Autodesk Inventor part; units mm, degrees
ref_plane "YZ Plane" through (0, 0, 0) normal (1, 0, 0) x (0, 1, 0)
ref_plane "XZ Plane" through (0, 0, 0) normal (0, 1, 0) x (-1, 0, 0)
ref_plane "XY Plane" through (0, 0, 0) normal (0, 0, 1) x (1, 0, 0)
sketch "Sketch1" plane through (0, 0, 0) normal (0, 0, 1) x (1, 0, 0)
  line L0 (-68.58, -128.7145) -> (68.58, -128.7145)
  line L1 (68.58, -128.7145) -> (68.58, 128.7145)
  line L2 (68.58, 128.7145) -> (-68.58, 128.7145)
  line L3 (-68.58, 128.7145) -> (-68.58, -128.7145)
  line L4 (-68.58, -128.7145) -> (68.58, 128.7145) construction
  line L5 (68.58, -128.7145) -> (-68.58, 128.7145) construction
  point P0 (0, 0)
  dimension "d0" = 137.16
  dimension "d1" = 257.429
extrude "Extrusion1" add sketch "Sketch1" against normal blind 3.175
sketch "Sketch2" plane through (0, 0, 0) normal (0, 0, 1) x (1, 0, 0)
  circle A0 centre (-59.69, 52.5145) radius 2.0955
  line L0 (-68.58, 128.7145) -> (-68.58, -128.7145)
  line L1 (-68.58, 128.7145) -> (68.58, 128.7145)
  circle A1 centre (59.69, 52.5145) radius 2.0955
  line L2 (68.58, -128.7145) -> (68.58, 128.7145)
  circle A2 centre (-59.69, -116.0145) radius 2.0955
  circle A3 centre (59.69, -116.0145) radius 2.0955
  line L3 (-68.58, -128.7145) -> (68.58, -128.7145)
  point P0 (0, 0)
  dimension "d4" = 8.89
  dimension "d5" = 76.2
  dimension "d6" = 76.2
  dimension "d7" = 8.89
  dimension "d8" = 4.191
  dimension "d9" = 12.7
  dimension "d10" = 8.89
  dimension "d11" = 8.89
  dimension "d12" = 12.7
  dimension "d13" = 4.191
  dimension "d21" = 4.191
  dimension "d22" = 4.191
hole "Hole1" at (-59.69, 52.5145, 0) at (59.69, 52.5145, 0) at (-59.69, -116.0145, 0) at (59.69, -116.0145, 0) direction (0, 0, -1) diameter 4.191 end through all
sketch "Sketch4" plane through (0, 0, 0) normal (0, 0, 1) x (1, 0, 0)
  line L0 (-35.179, -49.0855) -> (-35.179, -99.8855)
  line L1 (-28.321, -49.0855) -> (-28.321, -99.8855)
  line L2 (28.321, -49.0855) -> (28.321, -99.8855)
  line L3 (35.179, -49.0855) -> (35.179, -99.8855)
  line L4 (-68.58, 128.7145) -> (-68.58, -128.7145)
  line L5 (68.58, -128.7145) -> (68.58, 128.7145)
  line L6 (-68.58, -128.7145) -> (68.58, -128.7145)
  arc A0 (-28.321, -49.0855) -> (-35.179, -49.0855) centre (-31.75, -49.0855) ccw
  arc A1 (-35.179, -99.8855) -> (-28.321, -99.8855) centre (-31.75, -99.8855) ccw
  arc A2 (35.179, -49.0855) -> (28.321, -49.0855) centre (31.75, -49.0855) ccw
  arc A3 (28.321, -99.8855) -> (35.179, -99.8855) centre (31.75, -99.8855) ccw
  point P0 (0, 0)
  dimension "d23" = 6.858
  dimension "d24" = 6.858
  dimension "d25" = 33.401
  dimension "d26" = 50.8
  dimension "d27" = 33.401
  dimension "d28" = 28.829
  dimension "d29" = 28.829
  dimension "d30" = 28.829
  dimension "d31" = 28.829
  dimension "d32" = 50.8
  dimension "d33" = 50.8
  dimension "d34" = 50.8
extrude "Extrusion2" cut sketch "Sketch4" against normal blind 3.175
sketch "Sketch5" plane through (0, 0, 0) normal (0, 0, 1) x (1, 0, 0)
  line L0 (-68.58, 128.7145) -> (68.58, 128.7145)
  line L1 (68.58, 128.7145) -> (68.58, -128.7145)
  point P0 (0, 0)
  point P1 (-43.3324, 96.9645)
  point P2 (43.3324, 96.9645)
  dimension "d37" = 31.75
  dimension "d38" = 86.6648
  dimension "d39" = 31.75
  dimension "d40" = 25.2476
hole "Hole2" at (-43.3324, 96.9645, 0) at (43.3324, 96.9645, 0) direction (0, 0, -1) diameter 4.4704 end through all
sketch "battery_buzzer" plane through (0, 0, 0) normal (0, 0, 1) x (1, 0, 0)
  point P0 (0, 0)
sketch "Sketch10" plane through (0, 0, 0) normal (0, 0, 1) x (1, 0, 0)
  line L0 (-50.8, -128.7145) -> (-50.8, 39.8145)
  line L1 (-50.8, 39.8145) -> (50.8, 39.8145)
  line L2 (50.8, 39.8145) -> (50.8, -128.7145)
  line L3 (68.58, 128.7145) -> (-68.58, 128.7145)
  line L4 (-68.58, 128.7145) -> (-68.58, -128.7145)
  line L5 (68.58, 128.7145) -> (68.58, -128.7145)
  line L6 (-50.8, -128.7145) -> (50.8, -128.7145)
  point P0 (0, 0)
  dimension "d48" = 88.9
  dimension "d49" = 17.78
  dimension "d50" = 17.78
extrude "Extrusion3" cut sketch "Sketch10" against normal blind 3.175
CAD build for the part. Positions are in the model's coordinates, mm. Coordinates: 2 decimals unless noted, no trailing zeros. Write each loop counter-clockwise with the first axis right and the second up, starting at its lowest first coordinate (ties: lowest second). Pieces come first, ordered by that corner, then holes. Notation, with made-up numbers: M 80,63 L 130,63 A18 ccw 130,81 Z; hole C -24,43 d2. An arc over 180 degrees is marked long. Return JSON: item names as keys, results as strings.
Item 1: Two-plate mould, pull along X, no slides. Class faces 1 (the cylindrical face through (-45.549, 97.255, -1.61)), 2 (the flat face through (-1, 59, -3.175)): +X half, -X half, draft (parallel to the pull), parting line (faces both ways), or undercut.
Findings below:
{"face 1": "undercut", "face 2": "draft"}
Item 2: Drop flat-ended pins along their axis: pin 1 Ø4 at (x, y) = (-43.33, 96.96) entering from +Z; pin 2 Ø1 at (x, z) = (8, -1.5) entering from -Y. Give the stop position or say it passes through.
Findings below:
{"pin 1": "passes through", "pin 2": "stops at y = 39.81"}
Item 3: Slice it at C-C, the plane x = -35. Write the cut outline in (y, z) (1 decimal).
Findings below:
{"outline": "M 39.8,-3.2 L 128.7,-3.2 L 128.7,0 L 39.8,0 Z"}
Item 4: Probe line 1 (Y direction, x = 59.69, z = -1.45); line 2 (X direction, y = -24.5, z = -0.55); line 3 (Y direction, x = 15, z = -1.85). List the from-to ranges inside material, lowest first. Write a range as from..to.
Findings below:
{"line 1": "y = -128.71..-118.11, -113.92..50.42, 54.61..128.71", "line 2": "x = -68.58..-50.8, 50.8..68.58", "line 3": "y = 39.81..128.71"}
Item 5: Slice it at B-B, the plane z = -2.35. Write the cut outline in (x, y), and give its area (3 significant figures).
Findings below:
{"outline": "M -68.58,-128.71 L -50.8,-128.71 L -50.8,39.81 L 50.8,39.81 L 50.8,-128.71 L 68.58,-128.71 L 68.58,128.71 L -68.58,128.71 Z; hole C -59.69,-116.01 d4.19; hole C -59.69,52.51 d4.19; hole C -43.33,96.96 d4.47; hole C 43.33,96.96 d4.47; hole C 59.69,-116.01 d4.19; hole C 59.69,52.51 d4.19", "area": "18,100 mm2"}
Item 6: Slice it at A-A, the plane y = -57. Write the cut outline in (x, z) (3 decimals).
Findings below:
{"outline": "M -68.58,-3.175 L -50.8,-3.175 L -50.8,0 L -68.58,0 Z; M 50.8,-3.175 L 68.58,-3.175 L 68.58,0 L 50.8,0 Z"}
